from build123d import *

# Parameters (mm, degrees)
F0_W     = 50.8
F0_H     = 50.8
F1_DEPTH = 50.8
F2_R     = 6.35
F3_DEPTH = 50.801
F4_R     = 5.08
F5_R     = 5.08
F6_R     = 5.08
F7_R     = 5.08
F8_R     = 5.08


with BuildPart() as f1:
    # F0 (on Front) → F1 (new body)
    with BuildSketch(Plane.XZ):
        Rectangle(F0_W, F0_H)
    extrude(amount=F1_DEPTH)

    # F2 (on face) → F3 (cut, through all)
    with BuildSketch(Plane(origin=(0, 0, 0), x_dir=(-1, 0, 0), z_dir=(0, 1, 0))):
        Circle(F2_R)
        with Locations((12.7, -12.7)):
            Circle(F2_R)
        with Locations((-12.7, 12.7)):
            Circle(F2_R)
    extrude(amount=-F3_DEPTH, mode=Mode.SUBTRACT)

    # F4
    f4_edges = [f1.edges().sort_by_distance(p)[0] for p in [
        (-25.4, -25.4, 25.4),
    ]]
    fillet(f4_edges, radius=F4_R)

    # F5
    f5_edges = [f1.edges().sort_by_distance(p)[0] for p in [
        (-25.4, 0, -2.54),
    ]]
    fillet(f5_edges, radius=F5_R)

    # F6
    f6_edges = [f1.edges().sort_by_distance(p)[0] for p in [
        (-25.4, -50.8, -2.54),
    ]]
    fillet(f6_edges, radius=F6_R)

    # F7
    f7_edges = [f1.edges().sort_by_distance(p)[0] for p in [
        (-25.4, -25.4, -25.4),
    ]]
    fillet(f7_edges, radius=F7_R)

    # F8
    f8_edges = [f1.edges().sort_by_distance(p)[0] for p in [
        (25.4, 0, 0),
    ]]
    fillet(f8_edges, radius=F8_R)


solid = f1.part
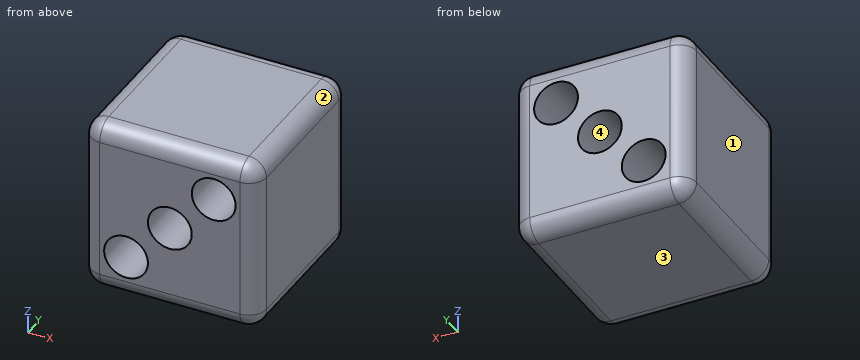
Design review of the part built by this model. Coordinates are the model's own, in mm. Face numbers are marked on the shaded views. Round coordinates to 2 decimals unless told otherwise and drop trailing zeros. Loops run counter-clockwise (first coordinate to the right, second up) from the corner with the lowest first, then second, coordinate; pieces in that order, holes last. Notation, with made-up numbers: (-17, 5) - (14, 5) arc R32 cw to (14, 40) - close; hole circle Ø11 at (12, -32.75). An arc over 180 degrees is marked (long way). One line per item, written item: value. Start each with the question number.
1) Consider section A-A on z = -12.7. Give the boundary of the cut face in (x, y), then the cut area to 3 significant figures.
2) Consider section B-B on x = -12.7. Give the boundary of the cut face in (y, z).
3) To check wall thickness, follow L1, parallel to Z at x = -12.7, y = -20; L2, parallel to Z at x = 13, y = -7; L3, parallel to X at y = -25, z = -12. State the ranges of each line that lie inside material, in increasing order. Write a range as from..to.
4) Insertion check: pin 1 Ø14.5 at (x, z) = (-12.7, -12.7) entering from -Y; pin 2 Ø10 at (x, z) = (12.7, 12.7) entering from +Y. Each pin has a flat end and moves straight along its axis. Give the tip position at first contact, or say it passes through.
5) Draft analysis for pull direction X (two halves, no side actions). For the marked faces 1, 2, 3 and 4, state which applies: +X half, -X half, draft (parallel to the pull), parting line (faces both ways), or undercut.
6) Consider section C-C on y = -45. Give the boundary of the cut face in (x, z).
Reported:
1. outline: (-25.4, -45.72) arc R5.08 ccw to (-20.32, -50.8) - (-19.05, -50.8) - (-19.05, 0) - (-20.32, 0) arc R5.08 ccw to (-25.4, -5.08) - close; (-6.35, -50.8) - (20.32, -50.8) arc R5.08 ccw to (25.4, -45.72) - (25.4, -5.08) arc R5.08 ccw to (20.32, 0) - (-6.35, 0) - close
1. area: 1,910 mm^2
2. outline: (-50.8, -20.32) arc R5.08 ccw to (-45.72, -25.4) - (-5.08, -25.4) arc R5.08 ccw to (0, -20.32) - (0, -19.05) - (-50.8, -19.05) - close; (-50.8, -6.35) - (0, -6.35) - (0, 20.32) arc R5.08 ccw to (-5.08, 25.4) - (-45.72, 25.4) arc R5.08 ccw to (-50.8, 20.32) - close
3. L1: z = -25.4..-19.05, -6.35..25.4
3. L2: z = -25.4..6.36, 19.04..25.4
3. L3: x = -25.4..-19.01, -6.39..25.4
4. pin 1: stops at y = -50.8
4. pin 2: passes through
5. face 1: -X half
5. face 2: +X half
5. face 3: draft
5. face 4: undercut
6. outline: (-25.4, -20.32) arc R5.08 ccw to (-20.32, -25.4) - (20.32, -25.4) arc R5.08 ccw to (25.4, -20.32) - (25.4, 20.32) arc R5.08 ccw to (20.32, 25.4) - (-20.32, 25.4) arc R5.08 ccw to (-25.4, 20.32) - close; hole circle Ø12.7 at (-12.7, -12.7); hole circle Ø12.7 at (0, 0); hole circle Ø12.7 at (12.7, 12.7)
